```python
from build123d import *

# Parameters (mm, degrees)
SKETCH1_W                = 41
SKETCH1_H                = 48
BOSS_EXTRUDE1_DEPTH      = 41
M2_CLEARANCE_HOLE1_D     = 2.459
M2_CLEARANCE_HOLE1_DEPTH = 4.5
FILLET1_R                = 2
FILLET2_R                = 0.5


with BuildPart() as part:
    # Sketch1 → Boss-Extrude1 (new body)
    with BuildSketch(Plane(origin=(0, 41, 0), x_dir=(1, 0, 0), z_dir=(0, 1, 0))):
        with Locations((-20.5, -24)):
            Rectangle(SKETCH1_W, SKETCH1_H)
    extrude(amount=-BOSS_EXTRUDE1_DEPTH)

    # Sketch2 → Revolve1 (revolve)
    with BuildSketch(Plane(origin=(0, 20.5, 0), x_dir=(1, 0, 0), z_dir=(0, 1, 0))):
        Polygon((-9.5, -48), (-20.5, -48), (-20.5, -72), (-18, -72), (-18, -50), (-9.5, -50), align=None)
    revolve(axis=Axis((-20.5, 20.5, 48), (0, 0, 1)))

    # M2 Clearance Hole1
    with Locations(Plane.XY.offset(48)):
        with Locations((-36.000338928, 4.999660985), (-5.000129304, 5.00012938), (-4.999606235, 36.000393851), (-35.999364901, 35.999364804)):
            Hole(M2_CLEARANCE_HOLE1_D / 2, depth=M2_CLEARANCE_HOLE1_DEPTH)

    # Fillet1
    fillet1_edges = [part.edges().sort_by_distance(p)[0] for p in [
        (0, 0, 24),
        (-41, 0, 24),
        (0, 41, 24),
        (-41, 41, 24),
    ]]
    fillet(fillet1_edges, radius=FILLET1_R)

    # Fillet2
    fillet2_edges = [part.edges().sort_by_distance(p)[0] for p in [
        (-20.5, 41, 0),
        (-41, 20.5, 0),
        (0, 20.5, 0),
        (-20.5, 0, 0),
        (-0.585786438, 0.585786438, 0),
        (-40.414213562, 0.585786438, 0),
        (-0.585786438, 40.414213562, 0),
        (-40.414213562, 40.414213562, 0),
    ]]
    fillet(fillet2_edges, radius=FILLET2_R)


solid = part.part
```
Geometry: final body of the model. Coordinates: model frame, mm. A direction names the side the tool comes from. Coordinates: 2 decimals unless noted, no trailing zeros. Loops run counter-clockwise (first coordinate to the right, second up) from the corner with the lowest first, then second, coordinate; pieces in that order, holes last. Notation, with made-up numbers: (89, -2.5) -> (117, -2.5) arc R12 ccw to (117, 11.5) -> close; hole circle Ø4 at (43, 53). An arc over 180 degrees is marked (long way). Use a Markdown table: item, result. Add a question column.
(1) Section query A-A, the plane y = 20.5. Return loops of the section in (x, z).
(2) Access query for faces 1 (the cylindrical face through (-34.77, 5.05, 45.72)), 2 (the flat face through (-20, 21, 72)). Directions: +Z, -Z, +X, -X, +Y, -Y. A direction counts if a zero-diameter tool reaches every point of the face in a straight line with its end or side. Return the directions, or none.
(3) Mould query, pull axis X, two halves, no side actions, for faces 3 (the cylindrical face through (-4.84, 37.22, 45.72)), 4 (the cylindrical face through (-40.43, 40.4, 23.92)), 5 (the cylindrical face through (-10.339, 16.287, 48.986)), 6 (the flat face through (-23, 18, 50)). Classes: pulls with the +X half, pulls with the -X half, needs draft (parallel to the pull), parting line crosses it, or undercut.
(4) Section query C-C, the plane y = 8. Return loops of the section in (x, z).
(5) Pin query (flat end, axial travel): pin 1 Ø2.5 at (x, y) = (-5.5, 4.5) entering from +Z; pin 2 Ø20.5 at (x, y) = (-16.5, 25.5) entering from +Z; pin 3 Ø0.7 at (x, y) = (-36, 36) entering from +Z; pin 4 Ø10 at (x, z) = (-16.5, 62) entering from +Y. Return the tip coordinate at first contact, or that it passes through.
(6) Section query D-D, the plane z = 61.5. Return loops of the section in (x, y).
(7) Line query: line 1 along Y through (x, z) = (-35.5, 44); line 2 along Z through (x, y) = (-37, 17); line 3 along Z through (x, y) = (-12.5, 27). Output: solid intervals per line, ascending.
(8) Section query B-B, the plane x = -20.5. Return loops of the section in (y, z).
Answer:
| question | item | result |
|---|---|---|
| 1 | outline | (-41, 0.5) arc R0.5 ccw to (-40.5, 0) -> (-0.5, 0) arc R0.5 ccw to (0, 0.5) -> (0, 48) -> (-9.5, 48) -> (-9.5, 50) -> (-18, 50) -> (-18, 72) -> (-23, 72) -> (-23, 50) -> (-31.5, 50) -> (-31.5, 48) -> (-41, 48) -> close |
| 2 | face 1 | +Z |
| 2 | face 2 | +Z, +X, -X, +Y, -Y |
| 3 | face 3 | undercut |
| 3 | face 4 | pulls with the -X half |
| 3 | face 5 | parting line crosses it |
| 3 | face 6 | needs draft |
| 4 | outline | (-41, 0.5) arc R0.5 ccw to (-40.5, 0) -> (-0.5, 0) arc R0.5 ccw to (0, 0.5) -> (0, 48) -> (-41, 48) -> close |
| 5 | pin 1 | stops at z = 48 |
| 5 | pin 2 | stops at z = 72 |
| 5 | pin 3 | stops at z = 43.5 |
| 5 | pin 4 | stops at y = 23 |
| 6 | outline | circle Ø5 at (-20.5, 20.5) |
| 7 | line 1 | y = 0 to 3.88, 6.12 to 34.88, 37.12 to 41 |
| 7 | line 2 | z = 0 to 48 |
| 7 | line 3 | z = 0 to 50 |
| 8 | outline | (0, 0.5) arc R0.5 ccw to (0.5, 0) -> (40.5, 0) arc R0.5 ccw to (41, 0.5) -> (41, 48) -> (31.5, 48) -> (31.5, 50) -> (23, 50) -> (23, 72) -> (18, 72) -> (18, 50) -> (9.5, 50) -> (9.5, 48) -> (0, 48) -> close |
